Can you work these out from the drawing? Everything is in mm from the part's minimum corner. Coordinates: 2 decimals unless noted, no trailing zeros. Order: outer loops, then holes, each group sorted by start corner. A loop starts at its lowest first (then second) coordinate and runs counter-clockwise, first axis right, second up. Notation, with made-up numbers: (-2, 34.5) - (11, 34.5) arc R24 cw to (11, 61.5) - close; hole circle Ø10 at (43.25, 2.25). An arc over 180 degrees is marked (long way). Answer as CSV lines item,"result". Start each with the question number.
Q1. Suppose I cut it at D-D (z = 13.75). Please give me the cut outline in (x, y) (1 decimal).
Q2. Suppose I cut it at B-B (z = 7.5). Please give me the cut outline in (x, y).
Q3. Suppose I cut it at C-C (y = 5.5). Please give me the cut outline in (x, z) (1 decimal).
Q4. For pin 1 Ø1 at (x, y) = (1.5, 9) entering from +Z; pin 2 Ø1.5 at (x, y) = (2, 5) entering from +Z, each with a flat end and sliding along its axis, tell me the tip position at first contact or that it passes through.
Q5. Suppose I cut it at A-A (x = 2.5). Count the separate pieces of the cut face and the enclosed holes in it.
Q6. I need wall thicknesses on line 1 (Z direction, x = 0.6, y = 3.75) (1 decimal); line 2 (Z direction, x = 1.05, y = 2.25) (1 decimal); line 3 (Y direction, x = 1.75, z = 7.75) (1 decimal). Which ranges of each line are inside material? Lowest first, please.
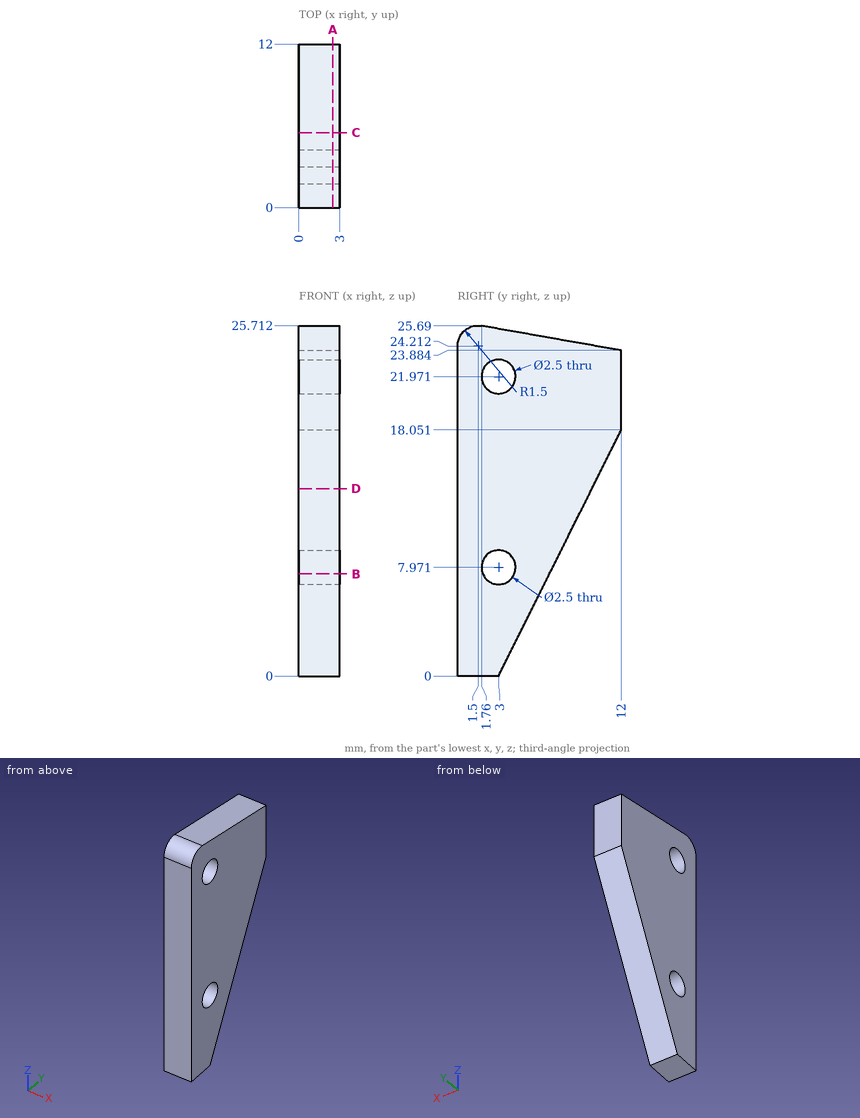
Here are the results:
1,outline,"(0, 0) - (3, 0) - (3, 9.9) - (0, 9.9) - close"
2,outline,"(0, 0) - (3, 0) - (3, 1.84) - (0, 1.84) - close; (0, 4.16) - (3, 4.16) - (3, 6.74) - (0, 6.74) - close"
3,outline,"(0, 5) - (3, 5) - (3, 25) - (0, 25) - close"
4,pin 1,"stops at z = 24.5"
4,pin 2,"stops at z = 25.25"
5,separate pieces,"1"
5,enclosed holes,"2"
6,line 1,"z = 1.5 to 7, 9 to 21, 23 to 25.3"
6,line 2,"z = 0 to 7, 9 to 21, 23 to 25.6"
6,line 3,"y = 0 to 1.8, 4.2 to 6.9"
